Source: CAD feature listing. Evaluate the final solid. Frame: model axes, mm. Coordinates: 2 decimals unless noted, no trailing zeros. Write each loop counter-clockwise with the first axis right and the second up, starting at its lowest first coordinate (ties: lowest second). Pieces come first, ordered by that corner, then holes. Notation, with made-up numbers: M 31,83.5 L 75,83.5 A21 ccw 75,113.5 Z; hole C -15,89 d6. An arc over 180 degrees is marked long. One line per item, written item: value. Start each with the question number.
Item 1: Cut plane A-A, the plane y = 0. Output: boundary loops of the cut face in (x, z), then the cut area to 3 significant figures.
Item 2: Cut plane C-C, the plane y = 26. Output: boundary loops of the cut face in (x, z) (1 decimal).
Item 3: Cut plane B-B, the plane x = -107.95. Output: boundary loops of the cut face in (y, z).
Item 4: Pin query (flat end, axial travel): P1, Ø5, axis at y = -17.5, z = 1, coming from the -X side; P2, Ø6, axis at x = -10.5, y = -5, coming from the -Z side; P3, Ø1, axis at y = 30, z = -1, coming from the +X side; P4, Ø3, axis at y = -9.5, z = 2, coming from the +X side. Return the tip coordinate at first contact, or that it passes through.
Item 5: Ray query, L1, parallel to Y at x = 107, z = 0.5; L2, parallel to X at y = -27.5, z = -1.25; L3, parallel to X at y = -11, z = -3. Return the intervals inside material, ascending. Write a range as from..to.
Item 6: Cut plane D-D, the plane x = 61.5. Output: boundary loops of the cut face in (y, z), then the cut area to 3 significant figures.
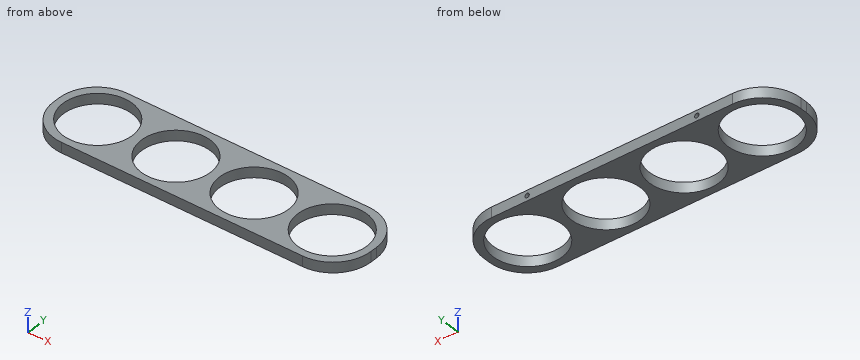
```python
from build123d import *

# Parameters (mm, degrees)
SKETCH1_W                  = 292.1
SKETCH1_H                  = 76.2
BOSS_EXTRUDE1_DEPTH        = 4.7625
SKETCH2_R                  = 31.75
CUT_EXTRUDE1_DEPTH         = 152.23801812
FILLET1_R                  = 34.925
F_10_32_TAPPED_HOLE2_D     = 4.0386
F_10_32_TAPPED_HOLE2_DEPTH = 19.05
F_10_32_TAPPED_HOLE2_TIP   = 1.213317848


with BuildPart() as part:
    # Sketch1 → Boss-Extrude1 (new, symmetric)
    with BuildSketch(Plane.XY):
        Rectangle(SKETCH1_W, SKETCH1_H)
    extrude(amount=BOSS_EXTRUDE1_DEPTH, both=True)

    # Sketch2 → Cut-Extrude1 (cut, through all)
    with BuildSketch(Plane.XY.offset(4.7625)):
        with Locations((-107.95, 0)):
            Circle(SKETCH2_R)
        with Locations((-35.983333333, 0)):
            Circle(SKETCH2_R)
        with Locations((35.983333333, 0)):
            Circle(SKETCH2_R)
        with Locations((107.95, 0)):
            Circle(SKETCH2_R)
    extrude(amount=-CUT_EXTRUDE1_DEPTH, mode=Mode.SUBTRACT)

    # Fillet1
    fillet1_edges = [part.edges().sort_by_distance(p)[0] for p in [
        (-146.05, 38.1, 0),
        (146.05, 38.1, 0),
        (146.05, -38.1, 0),
        (-146.05, -38.1, 0),
    ]]
    fillet(fillet1_edges, radius=FILLET1_R)

    # #10-32 Tapped Hole2
    with Locations(Plane(origin=(0, 38.1, 0), x_dir=(1, 0, 0), z_dir=(0, 1, 0))):
        with Locations((-78.105, 0), (78.105, 0)):
            Hole(F_10_32_TAPPED_HOLE2_D / 2, depth=F_10_32_TAPPED_HOLE2_DEPTH)
            with Locations((0, 0, -(F_10_32_TAPPED_HOLE2_DEPTH + F_10_32_TAPPED_HOLE2_TIP / 2))):  # 118° drill point
                Cone(0, F_10_32_TAPPED_HOLE2_D / 2, F_10_32_TAPPED_HOLE2_TIP, mode=Mode.SUBTRACT)


solid = part.part
```
From the geometry:
1. outline: M -146.05,-4.76 L -139.7,-4.76 L -139.7,4.76 L -146.05,4.76 Z; M -76.2,-4.76 L -67.73,-4.76 L -67.73,4.76 L -76.2,4.76 Z; M -4.23,-4.76 L 4.23,-4.76 L 4.23,4.76 L -4.23,4.76 Z; M 67.73,-4.76 L 76.2,-4.76 L 76.2,4.76 L 67.73,4.76 Z; M 139.7,-4.76 L 146.05,-4.76 L 146.05,4.76 L 139.7,4.76 Z
1. area: 363 mm²
2. outline: M -137.6,-4.8 L -126.2,-4.8 L -126.2,4.8 L -137.6,4.8 Z; M -89.7,-4.8 L -54.2,-4.8 L -54.2,4.8 L -89.7,4.8 Z; M -17.8,-4.8 L 17.8,-4.8 L 17.8,4.8 L -17.8,4.8 Z; M 54.2,-4.8 L 89.7,-4.8 L 89.7,4.8 L 54.2,4.8 Z; M 126.2,-4.8 L 137.6,-4.8 L 137.6,4.8 L 126.2,4.8 Z; hole C -78.1,0 d4; hole C 78.1,0 d4
3. outline: M -38.1,-4.76 L -31.75,-4.76 L -31.75,4.76 L -38.1,4.76 Z; M 31.75,-4.76 L 38.1,-4.76 L 38.1,4.76 L 31.75,4.76 Z
4. P1: stops at x = -143.99
4. P2: passes through
4. P3: stops at x = 134.08
4. P4: stops at x = 145.72
5. L1: y = -38.1..-31.74, 31.74..38.1
5. L2: x = -136.19..-123.82, -92.08..-51.85, -20.11..20.11, 51.85..92.08, 123.82..136.19
5. L3: x = -145.16..-137.73, -78.17..-65.77, -6.2..6.2, 65.77..78.17, 137.73..145.16
6. outline: M -38.1,-4.76 L -18.89,-4.76 L -18.89,4.76 L -38.1,4.76 Z; M 18.89,-4.76 L 38.1,-4.76 L 38.1,4.76 L 18.89,4.76 Z
6. area: 366 mm²
